Read the model definition and answer for the solid it produces. Units are mm, in the model's axes. A direction names the side the tool comes from. Coordinates: 2 decimals unless noted, no trailing zeros. Write each loop counter-clockwise with the first axis right and the second up, starting at its lowest first coordinate (ties: lowest second). Pieces come first, ordered by that corner, then holes. Notation, with made-up numbers: (-5.75, 42) -> (17.25, 42) arc R28 cw to (17.25, 79) -> close; hole circle Ø6 at (-7, -33). An arc over 180 degrees is marked (long way). Answer in a Markdown table with one row per item. Add a question column.
Item 1: Straight lines are drawn through the part: line 1 (Y direction, x = 0.25, z = -14.5); line 2 (Z direction, x = -3, y = -1.5); line 3 (Z direction, x = 0, y = -15.65). For each, find the intervals that lie inside material, in ascending order. Write a range as from..to.
Item 2: Section A-A on y = -5.25 is taken. Write down the section's boundary in (x, z), then the cut area to 3 significant figures.
Item 3: Given pin 1 Ø2.5 at (x, z) = (0.5, -10) entering from +Y; pin 2 Ø1.5 at (x, y) = (3, -3.5) entering from -Z; pin 3 Ø6 at (y, z) = (-4, -14) entering from +X, each flat-ended and moving along its own axis, determine where each tip first touches the part or whether it passes through.
Item 4: Section B-B on z = -20.5 is taken. Write down the section's boundary in (x, y), then the cut area to 3 significant figures.
Item 5: Which of the six approach directions +Z, -Z, +X, -X, +Y, -Y give full straight-line access (tool end or side, diameter ignored) to faces 4 (the face through (0.06, -2.99, -2.38)), 5 (the face through (0.056, -6.077, -17.769)), 6 (the face through (-3.553, -15.938, -5.462))?
Item 6: For a pull along Y with two mould halves and no side action, classify faces 1 (the face through (-3.969, -10, -5)), 2 (the face through (0.056, -12.831, -20.593)), 3 (the face through (0.06, -16.18, 3.07)) as +Y half, -Y half, draft (parallel to the pull), parting line (faces both ways), or undercut.
```python
from build123d import *

# Parameters (mm, degrees)
F1_DEPTH = 3.96875
F3_D     = 7.112
F3_DEPTH = 1.27
F3_TIP   = 2.1366603613
F4_D     = 0.79375
F4_DEPTH = 6.35
F4_START = 1.7053071
F4_TIP   = 0.2384665582


with BuildPart() as f1:
    # F0 (on Right) → F1 (new body, symmetric)
    with BuildSketch(Plane.YZ):
        with BuildLine():
            ThreePointArc((-16.5820843466, -28.1687893691), (-12.7313500896, -20.5184081186), (-4.2926705349, -19.0537665343))
            ThreePointArc((-4.2926705349, -19.0537665343), (-6.0968895961, -17.7448451986), (-7.0416428507, -15.7259537276))
            Line((-7.0416428507, -15.7259537276), (-7.0416428507, -7.5320968079))
            Line((-7.0416428507, -7.5320968079), (-7.0835554391, -7.4335314032))
            ThreePointArc((-7.0835554391, -7.4335314032), (-2.909546262, -2.3362589898), (3.6604483792, -1.846658048))
            Line((3.6604483792, -1.846658048), (6.0898731954, 2.6299539005))
            ThreePointArc((6.0898731954, 2.6299539005), (5.9660197938, 2.6908408891), (5.8412454606, 2.7498176323))
            Line((5.8412454606, 2.7498176323), (5.4112701147, 2.4430661607))
            Line((5.4112701147, 2.4430661607), (5.3323597714, 2.9668079517))
            ThreePointArc((5.3323597714, 2.9668079517), (5.1993250581, 3.0175413287), (5.0655028414, 3.0661594818))
            Line((5.0655028414, 3.0661594818), (4.6760486841, 2.7215427864))
            Line((4.6760486841, 2.7215427864), (4.5437401301, 3.2333209511))
            ThreePointArc((4.5437401301, 3.2333209511), (4.4049280258, 3.2719655055), (4.2655138361, 3.3083782172))
            Line((4.2655138361, 3.3083782172), (3.9063011974, 2.9300989368))
            Line((3.9063011974, 2.9300989368), (3.7280245356, 3.4267729314))
            ThreePointArc((3.7280245356, 3.4267729314), (3.587642111, 3.4520611622), (3.4468757875, 3.4751167886))
            Line((3.4468757875, 3.4751167886), (3.1119610132, 3.0673169038))
            Line((3.1119610132, 3.0673169038), (2.9009439477, 3.5430359177))
            ThreePointArc((2.9009439477, 3.5430359177), (2.8186697806, 3.5503399623), (2.7363319231, 3.5568870884))
            Line((2.7363319231, 3.5568870884), (2.4299388255, 3.115257909))
            Line((2.4299388255, 3.115257909), (2.1822380262, 3.5812106309))
            Line((2.1822380262, 3.5812106309), (1.9028896964, 3.5812106309))
            Line((1.9028896964, 3.5812106309), (1.6272033132, 3.1312487768))
            Line((1.6272033132, 3.1312487768), (1.3515187926, 3.5812106309))
            Line((1.3515187926, 3.5812106309), (1.0721187926, 3.5812106309))
            Line((1.0721187926, 3.5812106309), (0.7964324093, 3.1312487768))
            Line((0.7964324093, 3.1312487768), (0.5218389011, 3.5812106309))
            Line((0.5218389011, 3.5812106309), (-15.7920872965, 3.5812106309))
            Line((-15.7920872965, 3.5812106309), (-16.5820843466, 2.5423362134))
            Line((-16.5820843466, 2.5423362134), (-16.5820843466, -28.1687893691))
        make_face()
    extrude(amount=F1_DEPTH, both=True)

    # F3
    with Locations(Plane.XZ.offset(16.5820843466)):
        with Locations((0, -5.3087893691)):
            Hole(F3_D / 2, depth=F3_DEPTH)
            with Locations((0, 0, -(F3_DEPTH + F3_TIP / 2))):  # 118° drill point
                Cone(0, F3_D / 2, F3_TIP, mode=Mode.SUBTRACT)

    # F4
    # its depths count from where the whole tool has entered the part; down to there all is cleared
    with Locations(Plane.XZ.offset(16.5820843466).offset(-F4_START)):
        with Locations((3.2284024637, -5.3087893691)):
            Hole(F4_D / 2, depth=F4_DEPTH)
            with Locations((0, 0, -(F4_DEPTH + F4_TIP / 2))):  # 118° drill point
                Cone(0, F4_D / 2, F4_TIP, mode=Mode.SUBTRACT)


solid = f1.part
```
Results below:
| question | item | result |
|---|---|---|
| 1 | line 1 | y = -16.58..-7.04 |
| 1 | line 2 | z = -1.76..3.58 |
| 1 | line 3 | z = -24.06..-8.86, -1.75..3.58 |
| 2 | outline | (-3.97, -18.82) -> (3.97, -18.82) -> (3.97, -18.53) -> (-3.97, -18.53) -> close; (-3.97, -4.14) -> (3.97, -4.14) -> (3.97, 3.58) -> (-3.97, 3.58) -> close |
| 2 | area | 63.6 mm2 |
| 3 | pin 1 | stops at y = -7.04 |
| 3 | pin 2 | stops at z = -3.21 |
| 3 | pin 3 | passes through |
| 4 | outline | (-3.97, -16.58) -> (3.97, -16.58) -> (3.97, -12.71) -> (-3.97, -12.71) -> close |
| 4 | area | 30.8 mm2 |
| 5 | face 4 | +X, -X |
| 5 | face 5 | +X, -X, +Y |
| 5 | face 6 | -Y |
| 6 | face 1 | draft |
| 6 | face 2 | undercut |
| 6 | face 3 | -Y half |
